```python
from build123d import *

# Parameters (mm, degrees)
SKETCH099_W      = 5
SKETCH099_H      = 5
EXTRUDE035_DEPTH = 5
SKETCH100_R      = 1.6
HOLE021_DEPTH    = 2.2
HOLE021_TIPS_R   = 1.6


with BuildPart() as part:
    # Sketch099 (on Face9 of Pocket017) → Extrude035 (new body)
    with BuildSketch(Plane.XZ.offset(16.37)):
        with Locations((4.5, 18.8)):
            Rectangle(SKETCH099_W, SKETCH099_H)
    extrude(amount=EXTRUDE035_DEPTH)

    # Sketch100 (on Face1 of Extrude035) → Hole021 (cut)
    with BuildSketch(Plane.XY.offset(21.3)):
        with Locations((4, -18.4)):
            Circle(SKETCH100_R)
    extrude(amount=-HOLE021_DEPTH, mode=Mode.SUBTRACT)

    # Hole021 tips → Hole021 tip 1 section 0
    with BuildSketch(Plane.XY.offset(19.1), mode=Mode.PRIVATE) as hole021_tip_1_s0:
        with Locations((4, -18.4)):
            Circle(HOLE021_TIPS_R)
    loft([hole021_tip_1_s0.sketch, Vertex(4, -18.4, 18.138623)], mode=Mode.SUBTRACT)


solid = part.part
```
For this review, take the finished solid that the model builds, in its own axes (mm). A direction names the side the tool comes from. Round coordinates to 2 decimals unless told otherwise and drop trailing zeros. Write each loop counter-clockwise with the first axis right and the second up, starting at its lowest first coordinate (ties: lowest second). Pieces come first, ordered by that corner, then holes. Notation, with made-up numbers: (59.5, 1.25) -> (81.5, 1.25) arc R13 cw to (81.5, 20.25) -> close; hole circle Ø11 at (45, -2). An arc over 180 degrees is marked (long way). One line per question, with ' | ' between items. Start each with the question number.
(1) Mouldability with a two-part tool opening along X and no side actions: class faces 1 (the face through (4.137, -18.185, 18.292)), 2 (the face through (2, -19, 19)), 3 (the face through (4, -19, 16.3)) as released by +X, released by -X, zero draft, split by the parting line, or undercut.
(2) Tool access review of faces 4 (the face through (4, -16.37, 19)), 5 (the face through (4, -20, 20)): name each direction out of +Z, -Z, +X, -X, +Y, -Y from which nothing blocks a thin tool from reaching the whole face with its end or side.
(3) For line 1 along Y through (x, z) = (4, 20.3); line 2 along Y through (x, z) = (4.4, 20.5); line 3 along X through (y, z) = (-18.7, 18.45), list the stretches that pass through material, from the lowest coordinate up. Write a range as from..to.
(4) Add section B-B, the plane z = 18.4. Write out the cut boundary in (x, y) (3 decimals), plus the area to 3 significant figures.
(5) Add section A-A, the plane z = 20.9. Write out the cut boundary in (x, y).
Answer list:
1) face 1: undercut | face 2: released by -X | face 3: zero draft
2) face 4: +Z, -Z, +X, -X, +Y | face 5: +Z
3) line 1: -21.37..-20, -16.8..-16.37 | line 2: -21.37..-19.95, -16.85..-16.37 | line 3: 2..3.58, 4.42..7
4) outline: (2, -21.37) -> (7, -21.37) -> (7, -16.37) -> (2, -16.37) -> close; hole circle Ø0.87 at (4, -18.4) | area: 24.4 mm²
5) outline: (2, -21.37) -> (7, -21.37) -> (7, -16.37) -> (2, -16.37) -> close; hole circle Ø3.2 at (4, -18.4)
